The listing builds one solid part. Answer for the finished solid, in the listing's coordinates (mm). Round coordinates to 2 decimals unless told otherwise and drop trailing zeros. Write each loop counter-clockwise with the first axis right and the second up, starting at its lowest first coordinate (ties: lowest second). Pieces come first, ordered by that corner, then holes. Notation, with made-up numbers: (36.25, 12.5) - (62.25, 12.5) arc R18 cw to (62.25, 23.5) - close; hole circle Ø6 at (-26, 8). An arc over 180 degrees is marked (long way). Return JSON: item names as keys, results as strings. Group by question number.
from build123d import *

# Parameters (mm, degrees)
SKETCH2_R           = 1.5
BOSS_EXTRUDE1_DEPTH = 1.75
BOSS_EXTRUDE2_DEPTH = 3
BOSS_EXTRUDE3_DEPTH = 0.5
SKETCH5_R           = 0.25
CUT_EXTRUDE1_DEPTH  = 4.5


with BuildPart() as part:
    # Sketch2 → Boss-Extrude1 (new body)
    with BuildSketch(Plane(origin=(0, 0, 0), x_dir=(1, 0, 0), z_dir=(0, 1, 0))):
        with BuildLine():
            Line((-16, 18), (16, 18))
            ThreePointArc((16, 18), (17.414213562, 17.414213562), (18, 16))
            Line((18, 16), (18, -16))
            ThreePointArc((18, -16), (17.414213562, -17.414213562), (16, -18))
            Line((16, -18), (-16, -18))
            ThreePointArc((-16, -18), (-17.414213562, -17.414213562), (-18, -16))
            Line((-18, -16), (-18, 16))
            ThreePointArc((-18, 16), (-17.414213562, 17.414213562), (-16, 18))
        make_face()
        with Locations((-15.25, 15.25)):
            Circle(SKETCH2_R, mode=Mode.SUBTRACT)
        with Locations((15.25, 15.25)):
            Circle(SKETCH2_R, mode=Mode.SUBTRACT)
        with Locations((15.25, -15.25)):
            Circle(SKETCH2_R, mode=Mode.SUBTRACT)
        with Locations((-15.25, -15.25)):
            Circle(SKETCH2_R, mode=Mode.SUBTRACT)
    extrude(amount=BOSS_EXTRUDE1_DEPTH)

    # Sketch3 → Boss-Extrude2 (add)
    with BuildSketch(Plane.XY.offset(18)):
        with BuildLine():
            Line((7.124530098, 1.75), (11.124530098, 1.75))
            Line((11.124530098, 1.75), (11.124530098, 2.99232659))
            ThreePointArc((11.124530098, 2.99232659), (11.065951454, 3.133747946), (10.924530098, 3.19232659))
            Line((10.924530098, 3.19232659), (10.595445321, 3.19232659))
            ThreePointArc((10.595445321, 3.19232659), (10.454023965, 3.250905233), (10.395445321, 3.39232659))
            Line((10.395445321, 3.39232659), (10.395445321, 3.55))
            ThreePointArc((10.395445321, 3.55), (10.336866677, 3.691421356), (10.195445321, 3.75))
            Line((10.195445321, 3.75), (7.993768929, 3.75))
            ThreePointArc((7.993768929, 3.75), (7.852347573, 3.691421356), (7.793768929, 3.55))
            Line((7.793768929, 3.55), (7.793768929, 3.39232659))
            ThreePointArc((7.793768929, 3.39232659), (7.735190286, 3.250905233), (7.593768929, 3.19232659))
            Line((7.593768929, 3.19232659), (7.324530098, 3.19232659))
            ThreePointArc((7.324530098, 3.19232659), (7.183108742, 3.133747946), (7.124530098, 2.99232659))
            Line((7.124530098, 2.99232659), (7.124530098, 1.75))
        make_face()
        with BuildLine():
            Line((7.993768929, 3.65), (10.195445321, 3.65))
            ThreePointArc((10.195445321, 3.65), (10.266155999, 3.620710678), (10.295445321, 3.55))
            Line((10.295445321, 3.55), (10.295445321, 3.39232659))
            ThreePointArc((10.295445321, 3.39232659), (10.383313287, 3.180194555), (10.595445321, 3.09232659))
            Line((10.595445321, 3.09232659), (10.924530098, 3.09232659))
            ThreePointArc((10.924530098, 3.09232659), (10.995240776, 3.063037268), (11.024530098, 2.99232659))
            Line((11.024530098, 2.99232659), (11.024530098, 1.85))
            Line((11.024530098, 1.85), (7.224530098, 1.85))
            Line((7.224530098, 1.85), (7.224530098, 2.99232659))
            ThreePointArc((7.224530098, 2.99232659), (7.25381942, 3.063037268), (7.324530098, 3.09232659))
            Line((7.324530098, 3.09232659), (7.593768929, 3.09232659))
            ThreePointArc((7.593768929, 3.09232659), (7.805900964, 3.180194555), (7.893768929, 3.39232659))
            Line((7.893768929, 3.39232659), (7.893768929, 3.55))
            ThreePointArc((7.893768929, 3.55), (7.923058251, 3.620710678), (7.993768929, 3.65))
        make_face(mode=Mode.SUBTRACT)
    extrude(amount=-BOSS_EXTRUDE2_DEPTH)

    # Sketch4 → Boss-Extrude3 (add)
    with BuildSketch(Plane(origin=(0, 0, 15), x_dir=(-1, 0, 0), z_dir=(0, 0, -1))):
        with BuildLine():
            Line((-7.124530098, 1.75), (-7.124530098, 2.99232659))
            ThreePointArc((-7.124530098, 2.99232659), (-7.183108742, 3.133747946), (-7.324530098, 3.19232659))
            Line((-7.324530098, 3.19232659), (-7.593768929, 3.19232659))
            ThreePointArc((-7.593768929, 3.19232659), (-7.735190286, 3.250905233), (-7.793768929, 3.39232659))
            Line((-7.793768929, 3.39232659), (-7.793768929, 3.55))
            ThreePointArc((-7.793768929, 3.55), (-7.852347573, 3.691421356), (-7.993768929, 3.75))
            Line((-7.993768929, 3.75), (-10.195445321, 3.75))
            ThreePointArc((-10.195445321, 3.75), (-10.336866677, 3.691421356), (-10.395445321, 3.55))
            Line((-10.395445321, 3.55), (-10.395445321, 3.39232659))
            ThreePointArc((-10.395445321, 3.39232659), (-10.454023965, 3.250905233), (-10.595445321, 3.19232659))
            Line((-10.595445321, 3.19232659), (-10.924530098, 3.19232659))
            ThreePointArc((-10.924530098, 3.19232659), (-11.065951454, 3.133747946), (-11.124530098, 2.99232659))
            Line((-11.124530098, 2.99232659), (-11.124530098, 1.75))
            Line((-11.124530098, 1.75), (-7.124530098, 1.75))
        make_face()
    extrude(amount=BOSS_EXTRUDE3_DEPTH)

    # Sketch5 → Cut-Extrude1 (cut, through all)
    with BuildSketch(Plane(origin=(0, 0, 14.5), x_dir=(-1, 0, 0), z_dir=(0, 0, -1))):
        with Locations((-10.152838139, 2.618092042)):
            Circle(SKETCH5_R)
        with Locations((-9.352838139, 2.618092042)):
            Circle(SKETCH5_R)
        with Locations((-8.552838139, 2.618092042)):
            Circle(SKETCH5_R)
    extrude(amount=-CUT_EXTRUDE1_DEPTH, mode=Mode.SUBTRACT)


solid = part.part
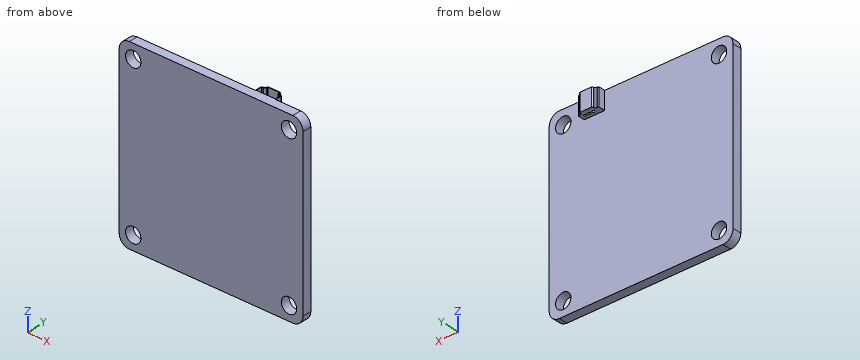
(1) Find section D-D (z = -2.5). Write down the section's boundary in (x, y), plus the area to 3 significant figures.
(2) Consider line 1 (X direction, y = 0.4, z = -15.25); line 2 (Z direction, x = 14.5, y = 1.7); line 3 (Y direction, x = -12.5, z = -1). Determine where each line is inside the solid, lowest interval first.
(3) Flat-ended cylindrical pins translate along their axes: pin 1 (1 mm diameter, centred on x = 10, y = 2.5, fed in from -Z); pin 2 (2 mm diameter, centred on x = 13.5, z = 4, fed in from +Y); pin 3 (2.5 mm diameter, centred on x = 15.25, z = 15.25, fed in from +Y); pin 4 (0.6 mm diameter, centred on y = 2.5, z = 16.5, fed in from -X). Find the tip coordinate at first contact, or state that the pin passes through.
(4) Find section C-C (x = -7). Write down the section's boundary in (y, z), plus the area to 3 significant figures.
(5) Find section B-B (y = 1.3). Write down the section's boundary in (x, z), plus the area to 3 significant figures.
(6) Find section A-A (x = -15.25). Write down the section's boundary in (y, z), plus the area to 3 significant figures.
Check sheet entries:
{
 "1": {"outline": "(-18, 0) - (18, 0) - (18, 1.75) - (-18, 1.75) - close", "area": "63.0 mm^2"},
 "2": {"line 1": "x = -18 to -16.75, -13.75 to 13.75, 16.75 to 18", "line 2": "z = -18 to -16.55, -13.95 to 13.95, 16.55 to 18", "line 3": "y = 0 to 1.75"},
 "3": {"pin 1": "stops at z = 14.5", "pin 2": "stops at y = 1.75", "pin 3": "passes through", "pin 4": "stops at x = 7.12"},
 "4": {"outline": "(0, -18) - (1.75, -18) - (1.75, 18) - (0, 18) - close", "area": "63.0 mm^2"},
 "5": {"outline": "(-18, -16) arc R2 ccw to (-16, -18) - (16, -18) arc R2 ccw to (18, -16) - (18, 16) arc R2 ccw to (16, 18) - (-16, 18) arc R2 ccw to (-18, 16) - close; hole circle Ø3 at (-15.25, -15.25); hole circle Ø3 at (-15.25, 15.25); hole circle Ø3 at (15.25, -15.25); hole circle Ø3 at (15.25, 15.25)", "area": "1,260 mm^2"},
 "6": {"outline": "(0, -18) - (1.75, -18) - (1.75, -16.75) - (0, -16.75) - close; (0, -13.75) - (1.75, -13.75) - (1.75, 13.75) - (0, 13.75) - close; (0, 16.75) - (1.75, 16.75) - (1.75, 18) - (0, 18) - close", "area": "52.5 mm^2"}
}
